Input: part model. Units: mm. Frame: model coordinates. Give positions to 0.01 mm unless a question says otherwise; leave off trailing zeros. Loops run counter-clockwise (first coordinate to the right, second up) from the corner with the lowest first, then second, coordinate; pieces in that order, holes last. Notation, with made-up numbers: (-34, 8.5) -> (-14, 8.5) arc R18 ccw to (-14, 15.5) -> close; hole circle Ø4 at (2.5, 60.25). An arc over 180 degrees is marked (long way). One line per question, with ' | ' between items.
from build123d import *

# Parameters (mm, degrees)
SKETCH1_W               = 319
SKETCH1_H               = 10
BOSS_EXTRUDE1_DEPTH     = 2
CUT_EXTRUDE1_DEPTH      = 160.590883198
CUT_EXTRUDE1_DEPTH_BACK = 160.590883198
SKETCH2_W               = 40
SKETCH2_H               = 2
CUT_EXTRUDE2_DEPTH      = 160.590883198
CUT_EXTRUDE2_DEPTH_BACK = 160.590883198
SKETCH4_W               = 2
SKETCH4_H               = 6


with BuildPart() as part:
    # Sketch1 → Boss-Extrude1 (new body)
    with BuildSketch(Plane(origin=(0, 0, 0), x_dir=(0, 0, -1), z_dir=(1, 0, 0))):
        Rectangle(SKETCH1_W, SKETCH1_H)
    extrude(amount=BOSS_EXTRUDE1_DEPTH)

    # Sketch2 → Cut-Extrude1 (cut, two sides: drawn at the far end of the back side and taken through both)
    with BuildSketch(Plane(origin=(2, 0, 0), x_dir=(0, 0, -1), z_dir=(1, 0, 0)).offset(-CUT_EXTRUDE1_DEPTH_BACK)):
        with Locations((-107.5, 4)):
            Rectangle(SKETCH2_W, SKETCH2_H)
        with Locations((-37.5, 4)):
            Rectangle(SKETCH2_W, SKETCH2_H)
        with Locations((37.5, 4)):
            Rectangle(SKETCH2_W, SKETCH2_H)
        with Locations((107.5, 4)):
            Rectangle(SKETCH2_W, SKETCH2_H)
    extrude(amount=CUT_EXTRUDE1_DEPTH + CUT_EXTRUDE1_DEPTH_BACK, mode=Mode.SUBTRACT)

    # Sketch4 → Cut-Extrude2 (cut, two sides: drawn at the far end of the back side and taken through both)
    with BuildSketch(Plane(origin=(2, 0, 0), x_dir=(0, 0, -1), z_dir=(1, 0, 0)).offset(-CUT_EXTRUDE2_DEPTH_BACK)):
        with Locations((1, 0)):
            Rectangle(SKETCH4_W, SKETCH4_H)
    extrude(amount=CUT_EXTRUDE2_DEPTH + CUT_EXTRUDE2_DEPTH_BACK, mode=Mode.SUBTRACT)


solid = part.part
1. Ray query, line 1 along Z through (x, y) = (0.9, 3.25); line 2 along Z through (x, y) = (0.3, 1.25); line 3 along Y through (x, z) = (1.35, 34.5). Return the intervals inside material, ascending. Write a range as from..to.
Determined:
line 1: z = -159.5..-127.5, -87.5..-57.5, -17.5..17.5, 57.5..87.5, 127.5..159.5 | line 2: z = -159.5..-2, 0..159.5 | line 3: y = -5..3
2. Section query A-A (x = 1.25). Output: boundary loops of the cut face in (y, z).
Determined:
outline: (-5, -159.5) -> (5, -159.5) -> (5, -127.5) -> (3, -127.5) -> (3, -87.5) -> (5, -87.5) -> (5, -57.5) -> (3, -57.5) -> (3, -17.5) -> (5, -17.5) -> (5, 17.5) -> (3, 17.5) -> (3, 57.5) -> (5, 57.5) -> (5, 87.5) -> (3, 87.5) -> (3, 127.5) -> (5, 127.5) -> (5, 159.5) -> (-5, 159.5) -> close; hole (-3, -2) -> (3, -2) -> (3, 0) -> (-3, 0) -> close
3. Section query B-B (z = 110.5). Output: boundary loops of the cut face in (x, y).
Determined:
outline: (0, -5) -> (2, -5) -> (2, 3) -> (0, 3) -> close
4. Pin query (flat end, axial travel): P1, Ø4, axis at y = 1.5, z = -92.5, coming from the -X side. Return the tip coordinate at first contact, or that it passes through.
Determined:
P1: stops at x = 0
